The listing builds one solid part. Answer for the finished solid, in the listing's coordinates (mm). A direction names the side the tool comes from. Coordinates: 2 decimals unless noted, no trailing zeros. Loops run counter-clockwise (first coordinate to the right, second up) from the corner with the lowest first, then second, coordinate; pieces in that order, holes last. Notation, with made-up numbers: (82.5, -23.75) -> (107.5, -23.75) arc R34 cw to (107.5, 10.25) -> close; hole circle Ø6 at (65, 58.5). An arc over 180 degrees is marked (long way). Answer in a Markdown table with one row per item.
```python
from build123d import *

# Parameters (mm, degrees)
EXTRUDE1_DEPTH                   = 2.5146
EXTRUDE1_DEPTH_BACK              = 2.5146
FILLET1_R                        = 2.5146
EXTRUDE2_DEPTH                   = 0.508
F_97_0_0059_DIAMETER_HOLE1_D     = 2.0574
F_97_0_0059_DIAMETER_HOLE1_DEPTH = 6.35


with BuildPart() as part:
    # Sketch1 → Extrude1 (new, two sides: drawn at the far end of the back side and taken through both)
    with BuildSketch(Plane(origin=(0, 0, 0), x_dir=(1, 0, 0), z_dir=(0, 1, 0)).offset(-EXTRUDE1_DEPTH_BACK)):
        with BuildLine():
            Line((-15.145893147, 13.572089242), (-15.145893147, 13.064089242))
            Line((-15.145893147, 13.064089242), (-15.112093192, 13.064089242))
            ThreePointArc((-15.112093192, 13.064089242), (-14.480623322, 12.844017507), (-14.122713826, 12.279140036))
            Line((-14.122713826, 12.279140036), (-12.14899346, 3.827499715))
            Line((-12.14899346, 3.827499715), (-11.654303777, 3.943025112))
            Line((-11.654303777, 3.943025112), (-13.628024142, 12.394665433))
            ThreePointArc((-13.628024142, 12.394665433), (-14.164888387, 13.24198164), (-15.112093192, 13.572089242))
            Line((-15.112093192, 13.572089242), (-15.145893147, 13.572089242))
        make_face()
    extrude(amount=EXTRUDE1_DEPTH + EXTRUDE1_DEPTH_BACK)

    # Fillet1
    fillet1_edges = [part.edges().sort_by_distance(p)[0] for p in [
        (-11.901648619, -2.5146, -3.885262414),
        (-11.901648619, 2.5146, -3.885262414),
    ]]
    fillet(fillet1_edges, radius=FILLET1_R - 0.0001)  # a hair under: the kernel refuses the full size

    # Sketch2 → Extrude2 (add)
    with BuildSketch(Plane(origin=(0, 0, -13.572089242), x_dir=(-1, 0, 0), z_dir=(0, 0, -1))):
        with BuildLine():
            Line((15.145893147, 2.5146), (15.145893147, -2.5146))
            Line((15.145893147, -2.5146), (16.267109258, -2.5146))
            ThreePointArc((16.267109258, -2.5146), (15.748, 0), (16.267109258, 2.5146))
            Line((16.267109258, 2.5146), (15.145893147, 2.5146))
        make_face()
    extrude(amount=-EXTRUDE2_DEPTH)

    # #97 (0.0059) Diameter Hole1
    with Locations(Plane(origin=(-12.191883936, 0, -6.244989577), x_dir=(0.227412198577, 0, 0.973798589), z_dir=(0.973798589, 0, -0.227412198577))):
        with Locations((0, 0)):
            Hole(F_97_0_0059_DIAMETER_HOLE1_D / 2, depth=F_97_0_0059_DIAMETER_HOLE1_DEPTH)


solid = part.part
```
Item 1: A cutting plane is placed at D-D, the plane z = -12.5. Determine the outline of the cut face in (x, y).
Findings below:
| item | result |
|---|---|
| outline | (-14.2, -2.51) -> (-13.66, -2.51) -> (-13.66, 2.51) -> (-14.2, 2.51) -> close |
Item 2: A cutting plane is placed at C-C, the plane y = -0.2. Determine the outline of the cut face in (x, z).
Findings below:
| item | result |
|---|---|
| outline | (-15.75, -13.57) -> (-15.11, -13.57) arc R1.52 ccw to (-13.63, -12.39) -> (-12.42, -7.23) -> (-12.92, -7.11) -> (-14.12, -12.28) arc R1.02 cw to (-15.11, -13.06) -> (-15.75, -13.06) -> close; (-12.46, -5.15) -> (-11.96, -5.26) -> (-11.66, -3.95) -> (-12.15, -3.84) -> close |
Item 3: A cutting plane is placed at B-B, the plane x = -15.3. Determine the outline of the cut face in (y, z), plus the area to 3 significant figures.
Findings below:
| item | result |
|---|---|
| outline | (-2.51, -13.57) -> (2.51, -13.57) -> (2.51, -13.06) -> (-2.51, -13.06) -> close |
| area | 2.55 mm2 |
Item 4: Flat-ended cylindrical pins translate along their axes: pin 1 Ø1 at (x, z) = (-14.5, -10) entering from -Y; pin 2 Ø0.9 at (x, y) = (-16, 1) entering from +Z; pin 3 Ø1.5 at (y, z) = (-2, -8) entering from +X; pin 4 Ø1 at (y, z) = (-1, -8.5) entering from -X. Find the tip coordinate at first contact, or state that the pin passes through.
Findings below:
| item | result |
|---|---|
| pin 1 | passes through |
| pin 2 | stops at z = -13.06 |
| pin 3 | stops at x = -12.43 |
| pin 4 | stops at x = -13.36 |
Item 5: A tool of negligible diameter and unlimited length cuts with its end or side. For faces 4 (the face through (-15.55, 0.04, -13.064)), 5 (the face through (-12.061, 1.758, -4.584)), from which of +Z, -Z, +X, -X, +Y, -Y can it reach the whole face along a straight path? Write none if from no direction.
Findings below:
| item | result |
|---|---|
| face 4 | +Z, -X, +Y, -Y |
| face 5 | +Z, +X, +Y |
Item 6: A cutting plane is placed at A-A, the plane y = -0.75. Determine the outline of the cut face in (x, z).
Findings below:
| item | result |
|---|---|
| outline | (-15.79, -13.57) -> (-15.11, -13.57) arc R1.52 ccw to (-13.63, -12.39) -> (-12.35, -6.93) -> (-12.85, -6.82) -> (-14.12, -12.28) arc R1.02 cw to (-15.11, -13.06) -> (-15.79, -13.06) -> close; (-12.53, -5.44) -> (-12.03, -5.56) -> (-11.68, -4.05) -> (-12.18, -3.94) -> close |
Item 7: Determine the mould class of faces 1 (the face through (-13.5, 2.515, -10.8)), 2 (the face through (-13.15, -0.04, -8.11)), 3 (the face through (-12.67, -0.31, -7.14)) for opening direction Y: +Y half, -Y half, draft (parallel to the pull), parting line (faces both ways), or undercut.
Findings below:
| item | result |
|---|---|
| face 1 | +Y half |
| face 2 | draft |
| face 3 | undercut |
Item 8: Find the intervals of material crossed by probe 1 along Y at (x, z) = (-12.15, -5.75); probe 2 along X at (y, z) = (2, -5); probe 3 along Z at (x, y) = (-15.2, -2), in increasing order.
Findings below:
| item | result |
|---|---|
| probe 1 | y = -2.43 to -0.9, 0.9 to 2.43 |
| probe 2 | x = -12.42 to -11.9 |
| probe 3 | z = -13.57 to -13.06 |
